Solid Edge part; units mm, degrees
sketch "Sketch1" plane through (0, 0, 0) normal (0, -1, 0) x (1, 0, 0)
  line L0 (19, 0) -> (19, 5)
  line L1 (19, 5) -> (22, 5)
  line L2 (22, 5) -> (22, 8.75)
  line L3 (22, 8.75) -> (7, 8.75)
  line L4 (7, 8.75) -> (7, 6)
  line L5 (7, 6) -> (0, 6)
  line L6 (0, 6) -> (0, 0)
  dimension "D1" = 19
  dimension "D2" = 7
revolve "RevolvedProtrusion1" add sketch "Sketch1" angle 360 about axis through (0, 0, 0) along (1, 0, 0)
hole "thread" at (19, 0, 0) direction (-1, 0, 0) diameter 4.7 depth 30 tip angle 118 start chamfer 0.4 start chamfer angle 45 end chamfer 0.4 end chamfer angle 45
chamfer "mounting_chamfers" distance 0.6 angle 45 2 edges at (0, 0, -6) (22, 0, -5)
properties material "Polyethylene, low density"
Check sheet for the modelled part. Datum: model origin and axes. Units: mm. A direction names the side the tool comes from. Round coordinates to 2 decimals unless told otherwise and drop trailing zeros. Loops run counter-clockwise (first coordinate to the right, second up) from the corner with the lowest first, then second, coordinate; pieces in that order, holes last.
1. Set-up check for faces 4 (the flat face through (7, 6, -2)), 5 (the cylindrical face through (20.22, 4.88, -1.08)), 6 (the flat face through (22, 6, 0)): record each of +Z, -Z, +X, -X, +Y, -Y from which the full face is reachable in a straight line by a thin tool's end or side.
2. Sectioned sample at A-A on y = 0. Record the boundary of the cut face in (x, z).
3. Scan lines: probe 1 along Y at (x, z) = (19.75, 0); probe 2 along Y at (x, z) = (14.75, 0). Record each from-to range of solid material in increasing order.
4. Gauge pin test, flat ends, axial feed: pin 1 Ø5 at (x, y) = (17.5, 7) entering from +Z; pin 2 Ø1.5 at (y, z) = (-2, -4.5) entering from -X; pin 3 Ø6 at (x, z) = (4.5, 3) entering from +Y; pin 4 Ø5 at (y, z) = (-1, 2) entering from +X. Record the tip position at first contact, or that the pin passes through.
5. Sectioned sample at C-C on x = 16.75. Record the boundary of the cut face in (y, z), and give its area (3 significant figures).
6. Sectioned sample at D-D on x = 5.75. Record the boundary of the cut face in (y, z).
7. Mould release check, pull along Z, two halves, no side actions. Record for faces 1 (the flat face through (0, 2.3, 2.3)), 2 (the flat face through (19, 2.2, 2.2)), 3 (the cylindrical face through (4, 0, -6)): released by +Z, released by -Z, zero draft, split by the parting line, or undercut.
Recorded:
1. face 4: -X
1. face 5: +X
1. face 6: +Z, -Z, +X, +Y, -Y
2. outline: (0, -5.4) - (0.6, -6) - (7, -6) - (7, -8.75) - (22, -8.75) - (22, -5.6) - (21.4, -5) - (19, -5) - (19, -2.75) - (18.6, -2.35) - (0.4, -2.35) - (0, -2.75) - close; (0, 2.75) - (0.4, 2.35) - (18.6, 2.35) - (19, 2.75) - (19, 5) - (21.4, 5) - (22, 5.6) - (22, 8.75) - (7, 8.75) - (7, 6) - (0.6, 6) - (0, 5.4) - close
3. probe 1: y = -8.75 to -5, 5 to 8.75
3. probe 2: y = -8.75 to -2.35, 2.35 to 8.75
4. pin 1: stops at z = 7.5
4. pin 2: stops at x = 0
4. pin 3: stops at y = 8.65
4. pin 4: stops at x = 19
5. outline: circle Ø17.5 at (0, 0); hole circle Ø4.7 at (0, 0)
5. area: 223 mm2
6. outline: circle Ø12 at (0, 0); hole circle Ø4.7 at (0, 0)
7. face 1: zero draft
7. face 2: undercut
7. face 3: split by the parting line
